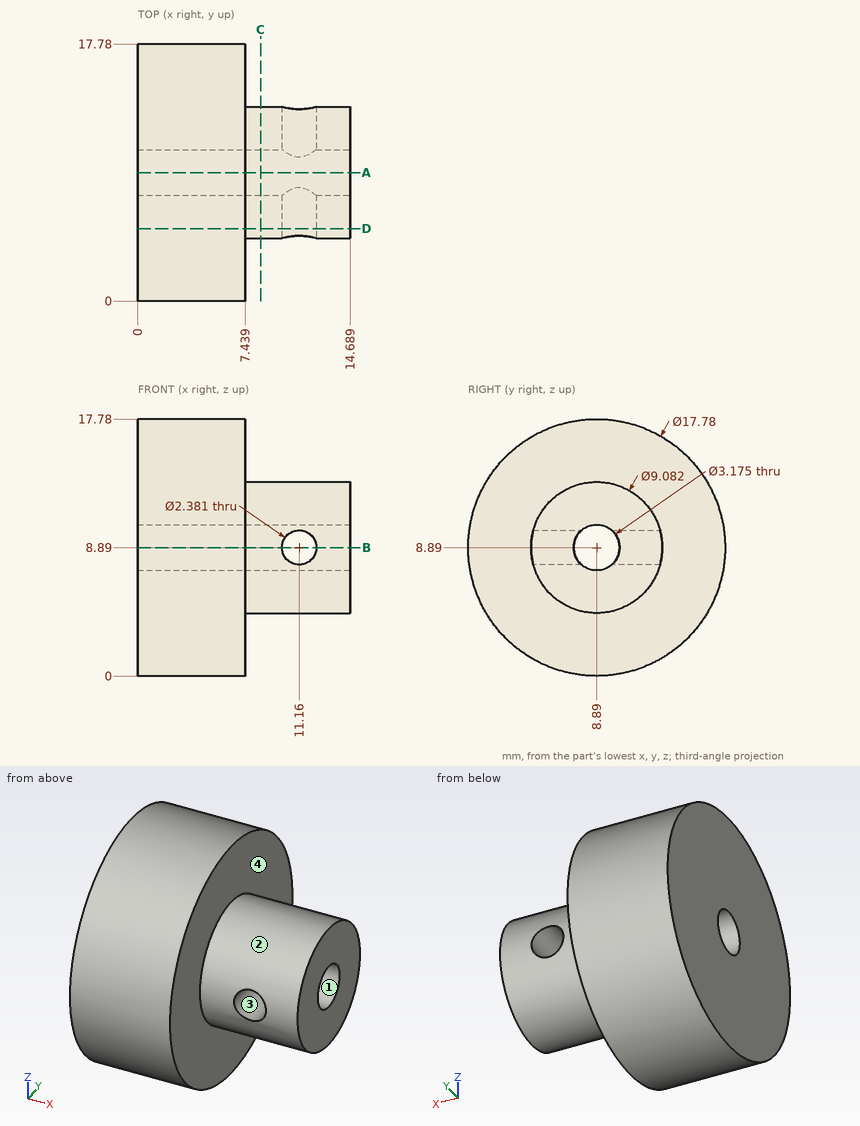
The drawing under review shows one solid part. Ordinate dimensions are in mm from its lowest x, y, z. Give positions to 0.01 mm unless a question says otherwise; leave off trailing zeros. Loops run counter-clockwise (first coordinate to the right, second up) from the corner with the lowest first, then second, coordinate; pieces in that order, holes last. Notation, with made-up numbers: M 4.5,41.25 L 49.5,41.25 A18 ccw 49.5,50.25 Z; hole C 57,31.5 d11. An arc over 180 degrees is marked long. Return JSON: item names as keys, results as strings. Group by question number.
Item 1: Insertion check: pin 1 Ø6 at (x, z) = (13, 5) entering from +Y; pin 2 Ø1.9 at (y, z) = (8.89, 8.89) entering from -X; pin 3 Ø4 at (x, z) = (11.16, 8.89) entering from -Y; pin 4 Ø1 at (y, z) = (4.5, 2) entering from +X. Each pin has a flat end and moves straight along its axis. Give the tip position at first contact, or say it passes through.
Item 2: We need section A-A (y = 8.89). Give the boundary of the cut face in (x, z).
Item 3: For probe 1 along Z at (x, y) = (8.25, 8.89); probe 2 along Z at (x, y) = (4, 9); probe 3 along X at (y, z) = (11.7, 8.89), list the stretches that pass through material, from the lowest coordinate up.
Item 4: We need section B-B (z = 8.89). Give the boundary of the cut face in (x, y).
Item 5: We need section D-D (y = 5). Give the boundary of the cut face in (x, z).
Item 6: Mouldability with a two-part tool opening along Z and no side actions: class the marked faces 1, 2, 3 and 4 as released by +Z, released by -Z, zero draft, split by the parting line, or undercut.
Item 7: We need section C-C (x = 8.5). Give the boundary of the cut face in (y, z) (1 decimal).
Output:
{
 "1": {"pin 1": "stops at y = 13.34", "pin 2": "passes through", "pin 3": "stops at y = 4.35", "pin 4": "stops at x = 7.44"},
 "2": {"outline": "M 0,0 L 7.44,0 L 7.44,4.35 L 14.69,4.35 L 14.69,7.3 L 0,7.3 Z; M 0,10.48 L 14.69,10.48 L 14.69,13.43 L 7.44,13.43 L 7.44,17.78 L 0,17.78 Z"},
 "3": {"probe 1": "z = 4.35 to 7.3, 10.48 to 13.43", "probe 2": "z = 0 to 7.31, 10.47 to 17.78", "probe 3": "x = 0 to 9.97, 12.35 to 14.69"},
 "4": {"outline": "M 0,0 L 7.44,0 L 7.44,4.35 L 9.97,4.35 L 9.97,7.3 L 0,7.3 Z; M 0,10.48 L 9.97,10.48 L 9.97,13.43 L 7.44,13.43 L 7.44,17.78 L 0,17.78 Z; M 12.35,4.35 L 14.69,4.35 L 14.69,7.3 L 12.35,7.3 Z; M 12.35,10.48 L 14.69,10.48 L 14.69,13.43 L 12.35,13.43 Z"},
 "5": {"outline": "M 0,0.9 L 7.44,0.9 L 7.44,6.55 L 14.69,6.55 L 14.69,11.23 L 7.44,11.23 L 7.44,16.88 L 0,16.88 Z; hole C 11.16,8.89 d2.38"},
 "6": {"face 1": "undercut", "face 2": "split by the parting line", "face 3": "undercut", "face 4": "zero draft"},
 "7": {"outline": "C 8.9,8.9 d9.1; hole C 8.9,8.9 d3.2"}
}
